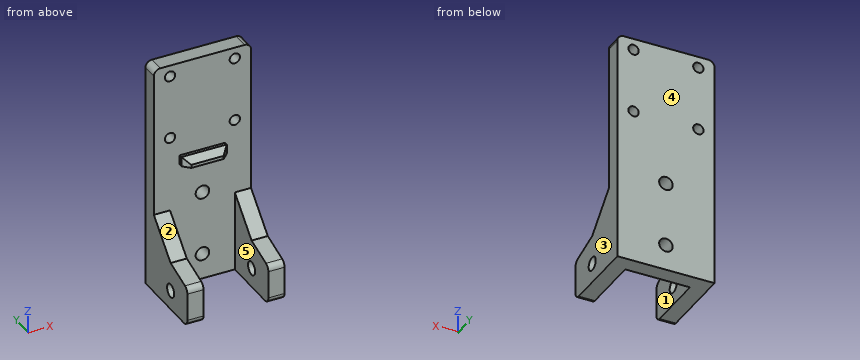
Autodesk Inventor part; units mm, degrees
ref_plane "YZ Plane" through (0, 0, 0) normal (1, 0, 0) x (0, 1, 0)
ref_plane "XZ Plane" through (0, 0, 0) normal (0, 1, 0) x (-1, 0, 0)
ref_plane "XY Plane" through (0, 0, 0) normal (0, 0, 1) x (1, 0, 0)
sketch "Sketch1" plane through (0, 0, 0) normal (0, 1, 0) x (-1, 0, 0)
  line L0 (15, 36) -> (-15, 36)
  line L1 (-15, 36) -> (-15, -36)
  line L2 (-15, -36) -> (15, -36)
  line L3 (15, -36) -> (15, 36)
  point P0 (0, 0)
  point P1 (0, 36)
  point P2 (15, 0)
  dimension "d0" = 30
  dimension "d1" = 72
extrude "Extrusion1" add sketch "Sketch1" along normal blind 5
sketch "Sketch2" plane through (0, 5, 0) normal (0, 1, 0) x (1, 0, 0)
  circle A0 centre (-10, -12.5) radius 1.6
  circle A1 centre (-10, -32.5) radius 1.6
  circle A2 centre (10, -32.5) radius 1.6
  circle A3 centre (10, -12.5) radius 1.6
  line L0 (-10, -32.5) -> (10, -32.5) construction
  line L1 (-15, -36) -> (15, -36)
  point P0 (0, 0)
  point P1 (0, -32.5)
  point P2 (0, -36)
  dimension "d4" = 3.2
  dimension "d5" = 20
  dimension "d6" = 20
  dimension "d7" = 3.5
extrude "Extrusion2" cut sketch "Sketch2" against normal up to next
sketch "Sketch3" plane through (0, 5, 0) normal (0, 1, 0) x (1, 0, 0)
  line L0 (15, 36) -> (-15, 36)
  circle A0 centre (0, 8) radius 2.1
  circle A1 centre (0, 28) radius 2.1
  point P0 (0, 0)
  point P1 (0, 36)
  point P2 (0, 36)
  point P3 (0, 36)
  point P4 (0, 36)
  point P5 (0, 36)
  dimension "d12" = 4.2
  dimension "d14" = 20
  dimension "d52" = 8
extrude "Extrusion3" cut sketch "Sketch3" against normal up to next
sketch "Sketch4" plane through (15, 0, 36) normal (1, 0, 0) x (0, 0, -1)
  line L0 (0, 0) -> (72, 0)
  line L1 (72, 0) -> (72, -20)
  line L2 (57, -10) -> (47, 0)
  line L3 (57, -10) -> (60, -20)
  line L4 (60, -20) -> (72, -20)
  line L5 (47, 0) -> (72, 0)
  point P0 (36, 0)
  point P1 (47, 5)
  point P2 (47, 5)
  point P3 (47, 5)
  dimension "d33" = 25
  dimension "d34" = 45
  dimension "d35" = 20
  dimension "d38" = 12
extrude "Extrusion4" add sketch "Sketch4" against normal blind 5
mirror "Mirror2" about plane through (0, 0, 0) normal (1, 0, 0) of "Extrusion4"
sketch "Sketch8" plane through (-15, 0, 36) normal (-1, 0, 0) x (0, 0, 1)
  circle A0 centre (-66, -10) radius 2.1
  line L0 (-60, -20) -> (-72, -20)
  point P0 (-36, 0)
  point P1 (-72, 0)
  point P2 (-66, -20)
  dimension "d39" = 4.2
  dimension "d40" = 10
extrude "Extrusion8" cut sketch "Sketch8" against normal through all
fillet "Fillet2" radius 2 6 edges at (-12.5, -20, -36) (-12.5, -20, -24) (12.5, -20, -24) (12.5, -20, -36) (-15, 2.5, 36) (15, 2.5, 36)
sketch "Sketch9" plane through (0, 0, 0) normal (0, -1, 0) x (1, 0, 0)
  line L0 (-7, 6) -> (7, 6)
  line L1 (7, 6) -> (7, 3)
  line L2 (7, 3) -> (-7, 3)
  line L3 (-7, 3) -> (-7, 6)
  line L4 (-13, 36) -> (13, 36)
  point P0 (0, 0)
  point P1 (0, 3)
  dimension "d44" = 33
  dimension "d45" = 3
  dimension "d46" = 14
extrude "Extrusion9" add sketch "Sketch9" along normal blind 3
chamfer "Chamfer1" distance 2 angle 45 3 edges at (-7, -3, 4.5) (0, -3, 6) (7, -3, 4.5)
ref_plane "Work Plane1" through (0, 0, 0) normal (1, 0, 0) x (0, 1, 0)
properties part number "X-connector-left"
The listing builds one solid part. Answer for the finished solid, in the listing's coordinates (mm). Face numbers are marked on the shaded views. A direction names the side the tool comes from. Round coordinates to 2 decimals unless told otherwise and drop trailing zeros. Loops run counter-clockwise (first coordinate to the right, second up) from the corner with the lowest first, then second, coordinate; pieces in that order, holes last. Notation, with made-up numbers: (7, -19) -> (13, -19) arc R23 cw to (13, 4) -> close; hole circle Ø10 at (-9, 55.25). An arc over 180 degrees is marked (long way). Use one line per item in the form item = value.
1. The part is cut by section D-D on x = 6. Determine the outline of the cut face in (y, z).
Answer key:
outline = (-2, 3) -> (0, 3) -> (0, -36) -> (5, -36) -> (5, 36) -> (0, 36) -> (0, 6) -> (-1, 6) -> (-2, 5) -> close
2. Flat-ended cylindrical pins translate along their axes: pin 1 Ø0.9 at (x, y) = (3, -1) entering from -Z; pin 2 Ø0.5 at (y, z) = (-0.5, 4.5) entering from -X; pin 3 Ø0.5 at (x, z) = (2, 3.5) entering from -Y. Find the tip coordinate at first contact, or state that the pin passes through.
Answer key:
pin_1 = 3
pin_2 = -7
pin_3 = -3
3. Find the intervals of material crossed by probe 1 along X at (y, z) = (2.1, 12.5); probe 2 along Y at (x, z) = (-11.2, -30); probe 3 along Z at (x, y) = (0, 3.2), in increasing order. Write a range as [from, to].
Answer key:
probe_1 = [-15, -11.6], [-8.4, 8.4], [11.6, 15]
probe_2 = [-20, -12.1], [-7.9, 5]
probe_3 = [-36, -30.1], [-25.9, -10.1], [-5.9, 36]
4. The part is cut by section B-B on x = 0. Determine the outline of the cut face in (y, z), and give its area (3 significant figures).
Answer key:
outline = (-3, 3) -> (0, 3) -> (0, -5.9) -> (5, -5.9) -> (5, 36) -> (0, 36) -> (0, 6) -> (-1, 6) -> (-3, 4) -> close; (0, -36) -> (5, -36) -> (5, -30.1) -> (0, -30.1) -> close; (0, -25.9) -> (5, -25.9) -> (5, -10.1) -> (0, -10.1) -> close
area = 325 mm²
5. The part is cut by section C-C on y = 0.75. Determine the outline of the cut face in (x, z), and give its area (3 significant figures).
Answer key:
outline = (-15, -36) -> (15, -36) -> (15, 34) arc R2 ccw to (13, 36) -> (-13, 36) arc R2 ccw to (-15, 34) -> close; hole circle Ø3.2 at (-10, 12.5); hole circle Ø3.2 at (-10, 32.5); hole circle Ø4.2 at (0, -28); hole circle Ø4.2 at (0, -8); hole circle Ø3.2 at (10, 12.5); hole circle Ø3.2 at (10, 32.5)
area = 2,100 mm²
6. The part is cut by section A-A on z = -8. Determine the outline of the cut face in (x, y).
Answer key:
outline = (-15, 0) -> (-2.1, 0) -> (-2.1, 5) -> (-15, 5) -> close; (2.1, 0) -> (15, 0) -> (15, 5) -> (2.1, 5) -> close
7. For a pull along X with two mould halves and no side action, classify the marked faces 1, 2 and 3 as released by +X, released by -X, zero draft, split by the parting line, or undercut.
Answer key:
face_1 = undercut
face_2 = zero draft
face_3 = released by +X
8. A tool of negligible diameter and unlimited length cuts with its end or side. For the marked faces 4 and 5, from which of +Z, -Z, +X, -X, +Y, -Y can it reach the whole face along a straight path? Write none if from no direction.
Answer key:
face_4 = +Z, -Z, +X, -X, +Y
face_5 = +Z, -Z, -Y
